```python
from build123d import *

# Parameters (mm, degrees)
BOSS_EXTRUDE1_DEPTH = 10


with BuildPart() as part:
    # Model → Boss-Extrude1 (new body)
    with BuildSketch(Plane.XY):
        Polygon((28.595430627, 208.079406788), (457.402364394, 208.079406788), (450.465147668, 265.002801404), (35.532647353, 265.002801404), align=None)
        with BuildLine():
            Line((395.310996933, 254.538077216), (206.313334547, 253.79734179))
            ThreePointArc((206.313334547, 253.79734179), (204.831877168, 253.726342411), (203.362371854, 253.525566384))
            ThreePointArc((203.362371854, 253.525566384), (201.915523421, 253.196404178), (200.503112299, 252.741637237))
            ThreePointArc((200.503112299, 252.741637237), (199.134879559, 252.164276657), (197.822433038, 251.469373641))
            ThreePointArc((197.822433038, 251.469373641), (196.574446388, 250.661348154), (195.401785154, 249.747432679))
            ThreePointArc((195.401785154, 249.747432679), (194.312018164, 248.73331433), (193.314718807, 247.628134658))
            ThreePointArc((193.314718807, 247.628134658), (192.416254629, 246.43882667), (191.624648452, 245.175873375))
            ThreePointArc((191.624648452, 245.175873375), (190.944865739, 243.847507192), (190.382926022, 242.465159548))
            ThreePointArc((190.382926022, 242.465159548), (189.942468925, 241.038153288), (189.627280625, 239.578356845))
            ThreePointArc((189.627280625, 239.578356845), (189.439494965, 238.096112854), (189.380672163, 236.603179306))
            ThreePointArc((189.380672163, 236.603179306), (189.451209877, 235.110754019), (189.65059371, 233.630026194))
            ThreePointArc((189.65059371, 233.630026194), (189.977255318, 232.172756129), (190.428843836, 230.749235263))
            ThreePointArc((190.428843836, 230.749235263), (191.001660076, 229.37136212), (191.691775805, 228.048337887))
            ThreePointArc((191.691775805, 228.048337887), (192.493322165, 226.791673876), (193.401016068, 225.609399465))
            ThreePointArc((193.401016068, 225.609399465), (194.406947639, 224.512071023), (195.504630226, 223.506525909))
            ThreePointArc((195.504630226, 223.506525909), (196.684373261, 222.601764862), (197.938701025, 221.803611967))
            ThreePointArc((197.938701025, 221.803611967), (199.256526594, 221.11895856), (200.629270456, 220.552399817))
            ThreePointArc((200.629270456, 220.552399817), (202.045191851, 220.108676612), (203.494586929, 219.790906907))
            ThreePointArc((203.494586929, 219.790906907), (204.965619617, 219.601640863), (206.447589253, 219.542270814))
            Line((206.447589253, 219.542270814), (395.445251639, 220.28300624))
            ThreePointArc((395.445251639, 220.28300624), (396.926709019, 220.354005619), (398.396214333, 220.554781645))
            ThreePointArc((398.396214333, 220.554781645), (399.843062766, 220.883943851), (401.255473887, 221.338710792))
            ThreePointArc((401.255473887, 221.338710792), (402.623706627, 221.916071373), (403.936153148, 222.610974389))
            ThreePointArc((403.936153148, 222.610974389), (405.184139798, 223.418999875), (406.356801033, 224.33291535))
            ThreePointArc((406.356801033, 224.33291535), (407.446568022, 225.347033699), (408.44386738, 226.452213372))
            ThreePointArc((408.44386738, 226.452213372), (409.342331557, 227.641521359), (410.133937735, 228.904474655))
            ThreePointArc((410.133937735, 228.904474655), (410.813720448, 230.232840838), (411.375660165, 231.615188482))
            ThreePointArc((411.375660165, 231.615188482), (411.816117262, 233.042194741), (412.131305562, 234.501991184))
            ThreePointArc((412.131305562, 234.501991184), (412.319091222, 235.984235175), (412.377914024, 237.477168724))
            ThreePointArc((412.377914024, 237.477168724), (412.30737631, 238.96959401), (412.107992477, 240.450321835))
            ThreePointArc((412.107992477, 240.450321835), (411.781330869, 241.9075919), (411.329742351, 243.331112767))
            ThreePointArc((411.329742351, 243.331112767), (410.756926111, 244.708985909), (410.066810382, 246.032010143))
            ThreePointArc((410.066810382, 246.032010143), (409.265264021, 247.288674153), (408.357570118, 248.470948564))
            ThreePointArc((408.357570118, 248.470948564), (407.351638547, 249.568277006), (406.253955961, 250.57382212))
            ThreePointArc((406.253955961, 250.57382212), (405.074212926, 251.478583167), (403.819885162, 252.276736063))
            ThreePointArc((403.819885162, 252.276736063), (402.502059592, 252.961389469), (401.129315731, 253.527948213))
            ThreePointArc((401.129315731, 253.527948213), (399.713394336, 253.971671417), (398.263999257, 254.289441123))
            ThreePointArc((398.263999257, 254.289441123), (396.792966569, 254.478707167), (395.310996933, 254.538077216))
        make_face(mode=Mode.SUBTRACT)
    extrude(amount=BOSS_EXTRUDE1_DEPTH)


solid = part.part
```
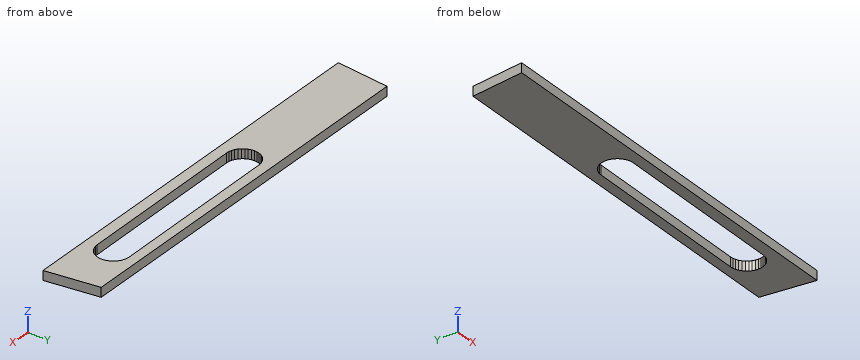
The listing builds one solid part. Answer for the finished solid, in the listing's coordinates (mm). Give positions to 0.01 mm unless a question says otherwise; leave off trailing zeros. Loops run counter-clockwise (first coordinate to the right, second up) from the corner with the lowest first, then second, coordinate; pieces in that order, holes last. Notation, with made-up numbers: M -5.75,77 L 10.25,77 A31 ccw 10.25,106 Z; hole C -33.75,-1 d8. An arc over 180 degrees is marked long. One line per item, written item: value.
Q1. A cutting plane is placed at B-B on y = 259. Determine the outline of the cut face in (x, z), then the cut area to 3 significant figures.
Working result:
outline: M 34.8,0 L 451.2,0 L 451.2,10 L 34.8,10 Z
area: 4,160 mm^2
Q2. Flat-ended cylindrical pins translate along their axes: P1, Ø6, axis at y = 235, z = 4, coming from the -X side; P2, Ø6, axis at y = 257, z = 5.5, coming from the +X side. Find the tip coordinate at first contact, or state that the pin passes through.
Working result:
P1: stops at x = 31.51
P2: stops at x = 451.81
Q3. A cutting plane is placed at A-A on x = 210. Determine the outline of the cut face in (y, z), then the cut area to 3 significant figures.
Working result:
outline: M 208.08,0 L 219.56,0 L 219.56,10 L 208.08,10 Z; M 253.81,0 L 265,0 L 265,10 L 253.81,10 Z
area: 227 mm^2
Q4. Find the intervals of material crossed by line 1 (Y direction, x = 227.5, z = 1.75); line 2 (Y direction, x = 266, z = 5.75); line 3 (X direction, y = 228.5, z = 8.25), in increasing order. Write a range as from..to.
Working result:
line 1: y = 208.08..219.62, 253.88..265
line 2: y = 208.08..219.78, 254.03..265
line 3: x = 31.08..191.44, 409.9..454.91
